```python
from build123d import *

# Parameters (mm, degrees)
SKETCH3_W           = 455.295
SKETCH3_H           = 277.368
BOSS_EXTRUDE1_DEPTH = 1.5875
CUT_EXTRUDE1_DEPTH  = 25.4


with BuildPart() as part:
    # Sketch3 → Boss-Extrude1 (new, symmetric)
    with BuildSketch(Plane.XY):
        Rectangle(SKETCH3_W, SKETCH3_H)
    extrude(amount=BOSS_EXTRUDE1_DEPTH, both=True)

    # Sketch4 → Cut-Extrude1 (cut)
    with BuildSketch(Plane.XY.offset(1.5875)):
        with BuildLine():
            Line((-161.29, 78.359001016), (-143.51, 78.359001016))
            ThreePointArc((-143.51, 78.359001016), (-139.917897552, 76.871103464), (-138.43, 73.279001016))
            Line((-138.43, 73.279001016), (-138.43, 32.639001016))
            ThreePointArc((-138.43, 32.639001016), (-139.917897552, 29.046898568), (-143.51, 27.559001016))
            Line((-143.51, 27.559001016), (-161.29, 27.559001016))
            ThreePointArc((-161.29, 27.559001016), (-164.882102448, 29.046898568), (-166.37, 32.639001016))
            Line((-166.37, 32.639001016), (-166.37, 73.279001016))
            ThreePointArc((-166.37, 73.279001016), (-164.882102448, 76.871103464), (-161.29, 78.359001016))
        make_face()
        with BuildLine():
            Line((-8.89, 78.359001016), (8.89, 78.359001016))
            ThreePointArc((8.89, 78.359001016), (12.482102448, 76.871103464), (13.97, 73.279001016))
            Line((13.97, 73.279001016), (13.97, 32.639001016))
            ThreePointArc((13.97, 32.639001016), (12.482102448, 29.046898568), (8.89, 27.559001016))
            Line((8.89, 27.559001016), (-8.89, 27.559001016))
            ThreePointArc((-8.89, 27.559001016), (-12.482102448, 29.046898568), (-13.97, 32.639001016))
            Line((-13.97, 32.639001016), (-13.97, 73.279001016))
            ThreePointArc((-13.97, 73.279001016), (-12.482102448, 76.871103464), (-8.89, 78.359001016))
        make_face()
        with BuildLine():
            Line((67.31, 78.359001016), (85.09, 78.359001016))
            ThreePointArc((85.09, 78.359001016), (88.682102448, 76.871103464), (90.17, 73.279001016))
            Line((90.17, 73.279001016), (90.17, 32.639001016))
            ThreePointArc((90.17, 32.639001016), (88.682102448, 29.046898568), (85.09, 27.559001016))
            Line((85.09, 27.559001016), (67.31, 27.559001016))
            ThreePointArc((67.31, 27.559001016), (63.717897552, 29.046898568), (62.23, 32.639001016))
            Line((62.23, 32.639001016), (62.23, 73.279001016))
            ThreePointArc((62.23, 73.279001016), (63.717897552, 76.871103464), (67.31, 78.359001016))
        make_face()
        with BuildLine():
            Line((143.51, 78.359001016), (161.29, 78.359001016))
            ThreePointArc((161.29, 78.359001016), (164.882102448, 76.871103464), (166.37, 73.279001016))
            Line((166.37, 73.279001016), (166.37, 32.639001016))
            ThreePointArc((166.37, 32.639001016), (164.882102448, 29.046898568), (161.29, 27.559001016))
            Line((161.29, 27.559001016), (143.51, 27.559001016))
            ThreePointArc((143.51, 27.559001016), (139.917897552, 29.046898568), (138.43, 32.639001016))
            Line((138.43, 32.639001016), (138.43, 73.279001016))
            ThreePointArc((138.43, 73.279001016), (139.917897552, 76.871103464), (143.51, 78.359001016))
        make_face()
        with BuildLine():
            Line((-85.09, 78.359001016), (-67.31, 78.359001016))
            ThreePointArc((-67.31, 78.359001016), (-63.717897552, 76.871103464), (-62.23, 73.279001016))
            Line((-62.23, 73.279001016), (-62.23, 32.639001016))
            ThreePointArc((-62.23, 32.639001016), (-63.717897552, 29.046898568), (-67.31, 27.559001016))
            Line((-67.31, 27.559001016), (-85.09, 27.559001016))
            ThreePointArc((-85.09, 27.559001016), (-88.682102448, 29.046898568), (-90.17, 32.639001016))
            Line((-90.17, 32.639001016), (-90.17, 73.279001016))
            ThreePointArc((-90.17, 73.279001016), (-88.682102448, 76.871103464), (-85.09, 78.359001016))
        make_face()
    extrude(amount=-CUT_EXTRUDE1_DEPTH, mode=Mode.SUBTRACT)


solid = part.part
```
CAD build for the part. Positions are in the model's coordinates, mm. Round coordinates to 2 decimals unless told otherwise and drop trailing zeros. Order: outer loops, then holes, each group sorted by start corner. A loop starts at its lowest first (then second) coordinate and runs counter-clockwise, first axis right, second up.
Q1. Wall check: L1, parallel to X at y = 41.5, z = 1.4; L2, parallel to Y at x = 85, z = 0.1; L3, parallel to X at y = 31, z = 0.8. Give the ranges that are in metal, low to high.
Q2. Slice it at A-A (x = 151). Write the cut outline in (y, z), and give its area (3 significant figures).
Q3. Slice it at B-B (y = 55). Write the cut outline in (x, z), and give its area (3 significant figures).
Q4. Slice it at C-C (z = 0.6). State how many separate pieces and enclosed holes the cut face has, and give its area (3 significant figures).
Results below:
1. L1: x = -227.65 to -166.37, -138.43 to -90.17, -62.23 to -13.97, 13.97 to 62.23, 90.17 to 138.43, 166.37 to 227.65
1. L2: y = -138.68 to 27.56, 78.36 to 138.68
1. L3: x = -227.65 to -166.1, -138.7 to -89.9, -62.5 to -13.7, 13.7 to 62.5, 89.9 to 138.7, 166.1 to 227.65
2. outline: (-138.68, -1.59) - (27.56, -1.59) - (27.56, 1.59) - (-138.68, 1.59) - close; (78.36, -1.59) - (138.68, -1.59) - (138.68, 1.59) - (78.36, 1.59) - close
2. area: 719 mm2
3. outline: (-227.65, -1.59) - (-166.37, -1.59) - (-166.37, 1.59) - (-227.65, 1.59) - close; (-138.43, -1.59) - (-90.17, -1.59) - (-90.17, 1.59) - (-138.43, 1.59) - close; (-62.23, -1.59) - (-13.97, -1.59) - (-13.97, 1.59) - (-62.23, 1.59) - close; (13.97, -1.59) - (62.23, -1.59) - (62.23, 1.59) - (13.97, 1.59) - close; (90.17, -1.59) - (138.43, -1.59) - (138.43, 1.59) - (90.17, 1.59) - close; (166.37, -1.59) - (227.65, -1.59) - (227.65, 1.59) - (166.37, 1.59) - close
3. area: 1,000 mm2
4. separate pieces: 1
4. enclosed holes: 5
4. area: 119,000 mm2
